Here's the drawing with two shaded views (mm, measured from the low corner). I have some questions. Give positions to 0.01 mm unless a question says otherwise; leave off trailing zeros. Write each loop counter-clockwise with the first axis right and the second up, starting at its lowest first coordinate (ties: lowest second). Pieces come first, ordered by that corner, then holes.
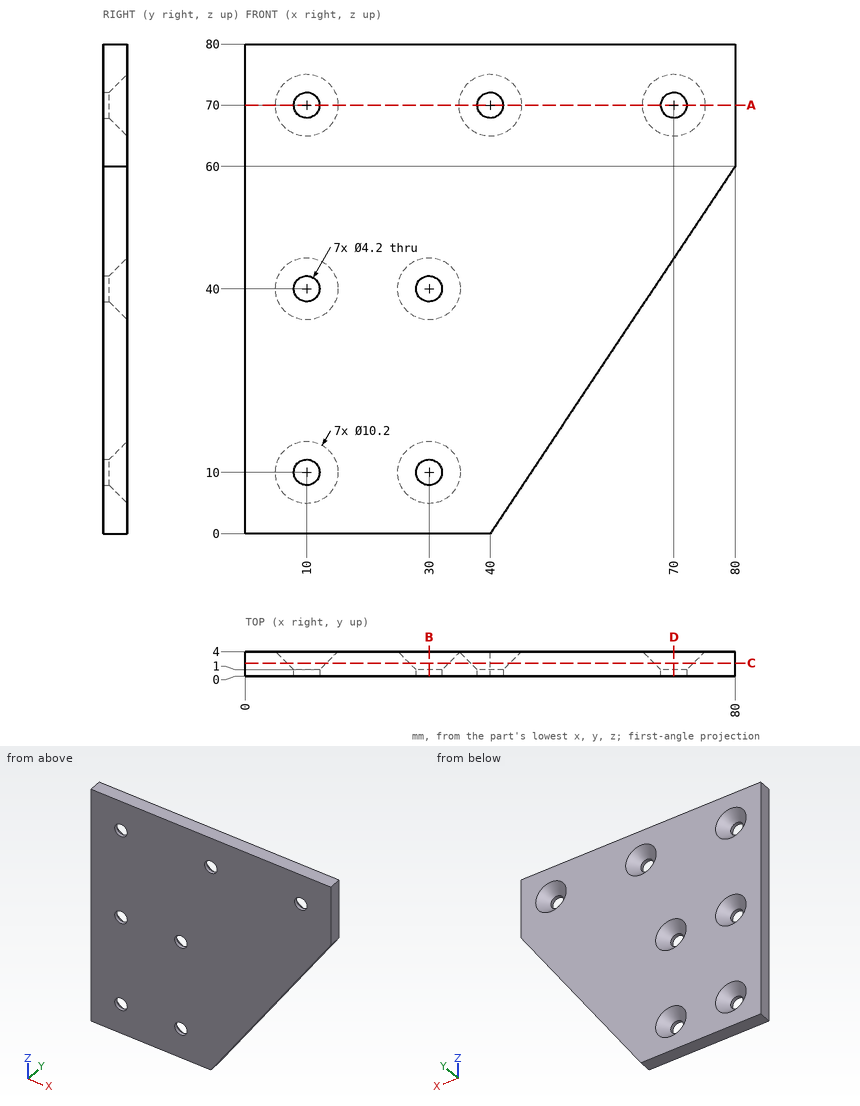
1) For pin 1 Ø5.5 at (x, z) = (40, 70) entering from -Y; pin 2 Ø6.5 at (x, z) = (10, 40) entering from +Y, each with a flat end and sliding along its axis, tell me the tip position at first contact or that it passes through.
Values follow:
pin 1: stops at y = 0
pin 2: stops at y = 2.15
2) Suppose I cut it at A-A on z = 70. Write out the boundary of the cut face in (x, y).
Values follow:
outline: (0, 0) - (7.9, 0) - (7.9, 1) - (4.9, 4) - (0, 4) - close; (12.1, 0) - (37.9, 0) - (37.9, 1) - (34.9, 4) - (15.1, 4) - (12.1, 1) - close; (42.1, 0) - (67.9, 0) - (67.9, 1) - (64.9, 4) - (45.1, 4) - (42.1, 1) - close; (72.1, 0) - (80, 0) - (80, 4) - (75.1, 4) - (72.1, 1) - close
3) Please list where these lines run through material, in increasing order: L1, parallel to Z at x = 30, y = 0.75; L2, parallel to X at y = 0.5, z = 70.
Values follow:
L1: z = 0 to 7.9, 12.1 to 37.9, 42.1 to 80
L2: x = 0 to 7.9, 12.1 to 37.9, 42.1 to 67.9, 72.1 to 80
4) Suppose I cut it at B-B on x = 30. Write out the boundary of the cut face in (y, z), plus the area to 3 significant figures.
Values follow:
outline: (0, 0) - (4, 0) - (4, 4.9) - (1, 7.9) - (0, 7.9) - close; (0, 12.1) - (1, 12.1) - (4, 15.1) - (4, 34.9) - (1, 37.9) - (0, 37.9) - close; (0, 42.1) - (1, 42.1) - (4, 45.1) - (4, 80) - (0, 80) - close
area: 268 mm2
5) Suppose I cut it at C-C on y = 2.1. Write out the boundary of the cut face in (x, z).
Values follow:
outline: (0, 0) - (40, 0) - (80, 60) - (80, 80) - (0, 80) - close; hole circle Ø6.4 at (10, 10); hole circle Ø6.4 at (10, 40); hole circle Ø6.4 at (10, 70); hole circle Ø6.4 at (30, 10); hole circle Ø6.4 at (30, 40); hole circle Ø6.4 at (40, 70); hole circle Ø6.4 at (70, 70)
6) Suppose I cut it at D-D on x = 70. Write out the boundary of the cut face in (y, z).
Values follow:
outline: (0, 45) - (4, 45) - (4, 64.9) - (1, 67.9) - (0, 67.9) - close; (0, 72.1) - (1, 72.1) - (4, 75.1) - (4, 80) - (0, 80) - close
